```python
from build123d import *

# Parameters (mm, degrees)
F0_W     = 101.6
F0_H     = 63.5
F1_DEPTH = 12.7
F2_R     = 6.35
F3_DEPTH = 12.701
F4_W     = 19.05
F4_H     = 38.1
F6_W     = 11.628822
F6_H     = 12.7


with BuildPart() as f1:
    # F0 (on Top) → F1 (new body)
    with BuildSketch(Plane.XY):
        Rectangle(F0_W, F0_H)
    extrude(amount=F1_DEPTH)

    # F2 (on face) → F3 (cut, through all)
    with BuildSketch(Plane.XY.offset(12.7)):
        with Locations((-38.1, 19.05)):
            Circle(F2_R)
        with Locations((-38.1, -21.987695)):
            Circle(F2_R)
        with Locations((38.1, 18.410703)):
            Circle(F2_R)
        with Locations((38.1, -20.573199)):
            Circle(F2_R)
    extrude(amount=-F3_DEPTH, mode=Mode.SUBTRACT)

    # F4 (on Front) → F5 (revolve)
    with BuildSketch(Plane.XZ):
        with Locations((-9.525, 31.75)):
            Rectangle(F4_W, F4_H)
    revolve(axis=Axis((0, 0, 31.75), (0, 0, -1)))

    # F6 (on Front) → F7 (revolve, cut)
    with BuildSketch(Plane.XZ):
        with Locations((-19.727555, 31.75)):
            Rectangle(F6_W, F6_H)
    revolve(axis=Axis((0, 0, 28.649839), (0, 0, 1)), mode=Mode.SUBTRACT)


solid = f1.part
```
The model under review builds one solid part; all positions refer to its coordinate system, in mm. A direction names the side the tool comes from. Round coordinates to 2 decimals unless told otherwise and drop trailing zeros. Order: outer loops, then holes, each group sorted by start corner. A loop starts at its lowest first (then second) coordinate and runs counter-clockwise, first axis right, second up. Notation, with made-up numbers: M 82,64.25 L 86,64.25 A23 ccw 86,75.25 Z; hole C 88,-35 d3. An arc over 180 degrees is marked long. Use a Markdown table: item, result.
1) Insertion check: pin 1 (10 mm diameter, centred on x = -6, z = 40.5, fed in from +Y); pin 2 (20.5 mm diameter, centred on x = -38.1, y = -21.99, fed in from +Z); pin 3 (5 mm diameter, centred on y = 0, z = 42, fed in from +X). Each pin has a flat end and moves straight along its axis. Give the tip position at first contact, or say it passes through.
Report:
| item | result |
|---|---|
| pin 1 | y = 19.02 |
| pin 2 | z = 12.7 |
| pin 3 | x = 19.05 |
2) Consider section D-D (y = 16). Write out the cut boundary in (x, z), then the cut area to 3 significant figures.
Report:
| item | result |
|---|---|
| outline | M -50.8,0 L -43.67,0 L -43.67,12.7 L -50.8,12.7 Z; M -32.53,0 L 32.23,0 L 32.23,12.7 L 10.34,12.7 L 10.34,25.4 L -10.34,25.4 L -10.34,12.7 L -32.53,12.7 Z; M -10.34,38.1 L 10.34,38.1 L 10.34,50.8 L -10.34,50.8 Z; M 43.97,0 L 50.8,0 L 50.8,12.7 L 43.97,12.7 Z |
| area | 1,520 mm^2 |
3) Consider section B-B (y = 0). Write out the cut boundary in (x, z).
Report:
| item | result |
|---|---|
| outline | M -50.8,0 L 50.8,0 L 50.8,12.7 L 19.05,12.7 L 19.05,25.4 L 13.91,25.4 L 13.91,38.1 L 19.05,38.1 L 19.05,50.8 L -19.05,50.8 L -19.05,38.1 L -13.91,38.1 L -13.91,25.4 L -19.05,25.4 L -19.05,12.7 L -50.8,12.7 Z |
4) Draft analysis for pull direction Y (two halves, no side actions). For faces 4 (the face through (33.061, -24.437, 6.439)), 5 (the face through (-1.32, 14.02, 25.4)), 6 (the face through (-1, -31.75, 6)), state which applies: released by +Y, released by -Y, zero draft, split by the parting line, or undercut.
Report:
| item | result |
|---|---|
| face 4 | undercut |
| face 5 | zero draft |
| face 6 | released by -Y |
5) Wall thickness on line 1 along Y through (x, z) = (-38.1, 4.5); line 2 along Y through (x, z) = (38, 3); line 3 along X through (y, z) = (-20, 11): over which ranges is each line inside the solid? List them lowest first. Write a range as [from, to].
Report:
| item | result |
|---|---|
| line 1 | [-31.75, -28.34], [-15.64, 12.7], [25.4, 31.75] |
| line 2 | [-31.75, -26.92], [-14.22, 12.06], [24.76, 31.75] |
| line 3 | [-50.8, -44.13], [-32.07, 31.78], [44.42, 50.8] |
6) Consider section C-C (z = 7). Write out the cut boundary in (x, y), then the cut area to 3 significant figures.
Report:
| item | result |
|---|---|
| outline | M -50.8,-31.75 L 50.8,-31.75 L 50.8,31.75 L -50.8,31.75 Z; hole C -38.1,-21.99 d12.7; hole C -38.1,19.05 d12.7; hole C 38.1,-20.57 d12.7; hole C 38.1,18.41 d12.7 |
| area | 5,940 mm^2 |
7) Consider section A-A (x = 38.1). Write out the cut boundary in (y, z), then the cut area to 3 significant figures.
Report:
| item | result |
|---|---|
| outline | M -31.75,0 L -26.92,0 L -26.92,12.7 L -31.75,12.7 Z; M -14.22,0 L 12.06,0 L 12.06,12.7 L -14.22,12.7 Z; M 24.76,0 L 31.75,0 L 31.75,12.7 L 24.76,12.7 Z |
| area | 484 mm^2 |
8) Tool access review of faces 1 (the face through (-32.043, 20.957, 6.439)), 2 (the face through (1.811, -13.795, 31.839)), 3 (the face through (15.12, -11.59, 19.14)): name each direction out of +Z, -Z, +X, -X, +Y, -Y from which nothing blocks a thin tool from reaching the whole face with its end or side.
Report:
| item | result |
|---|---|
| face 1 | +Z, -Z |
| face 2 | none |
| face 3 | +Z |
